from build123d import *

# Parameters (mm, degrees)
SKETCH1_W                     = 56
SKETCH1_H                     = 65
BOSS_EXTRUDE1_DEPTH           = 8
FILLET1_R                     = 3
CBORE_FOR_M4_SHCS1_AT_2_COUNT = 2
CBORE_FOR_M4_SHCS1_AT_2_PITCH = 24
M4X0_7_TAPPED_HOLE1_D         = 3.3
M4X0_7_TAPPED_HOLE1_DEPTH     = 10.1
M4X0_7_TAPPED_HOLE1_TIP       = 0.991420021


with BuildPart() as part:
    # Sketch1 → Boss-Extrude1 (new body)
    with BuildSketch(Plane.XY):
        Rectangle(SKETCH1_W, SKETCH1_H)
    extrude(amount=BOSS_EXTRUDE1_DEPTH)

    # Fillet1
    fillet1_edges = [part.edges().sort_by_distance(p)[0] for p in [
        (28, -32.5, 4),
        (-28, -32.5, 4),
        (-28, 32.5, 4),
        (28, 32.5, 4),
    ]]
    fillet(fillet1_edges, radius=FILLET1_R)

    # Sketch3 → CBORE for M4 SHCS1 (revolve, cut)
    with BuildSketch(Plane(origin=(-12, -22.5, 8), x_dir=(0, -1, 0), z_dir=(1, 0, 0))):
        Polygon((0, 0), (0, 8), (2.25, 8), (2.25, 4), (4, 4), (4, 0.025), (4.025, 0), align=None)
    cbore_for_m4_shcs1 = revolve(axis=Axis((-12, -22.5, 14.35), (0, 0, -1)), mode=Mode.SUBTRACT)

    # CBORE for M4 SHCS1 at 2: CBORE for M4 SHCS1 ×2
    with Locations(*[(i * CBORE_FOR_M4_SHCS1_AT_2_PITCH, 0, 0) for i in range(1, CBORE_FOR_M4_SHCS1_AT_2_COUNT)]):
        add(cbore_for_m4_shcs1, mode=Mode.SUBTRACT)

    # M4x0.7 Tapped Hole1
    with Locations(Plane.XY.offset(8)):
        with Locations((-23.25, -18.5), (23.25, -18.5), (23.25, 28), (-23.25, 28)):
            Hole(M4X0_7_TAPPED_HOLE1_D / 2, depth=M4X0_7_TAPPED_HOLE1_DEPTH)
            with Locations((0, 0, -(M4X0_7_TAPPED_HOLE1_DEPTH + M4X0_7_TAPPED_HOLE1_TIP / 2))):  # 118° drill point
                Cone(0, M4X0_7_TAPPED_HOLE1_D / 2, M4X0_7_TAPPED_HOLE1_TIP, mode=Mode.SUBTRACT)


solid = part.part
The model under review builds one solid part; all positions refer to its coordinate system, in mm. A direction names the side the tool comes from. Coordinates: 2 decimals unless noted, no trailing zeros. Loops run counter-clockwise (first coordinate to the right, second up) from the corner with the lowest first, then second, coordinate; pieces in that order, holes last.
(1) Tool access review of faces 4 (the cylindrical face through (-12.176, -18.504, 6.015)), 5 (the flat face through (28, 0, 4)): name each direction out of +Z, -Z, +X, -X, +Y, -Y from which nothing blocks a thin tool from reaching the whole face with its end or side.
Determined:
face 4: +Z
face 5: +Z, -Z, +X, +Y, -Y
(2) Consider section B-B, the plane x = -12. Give the boundary of the cut face in (y, z) (3 decimals).
Determined:
outline: (-32.5, 0) - (-24.75, 0) - (-24.75, 4) - (-26.5, 4) - (-26.5, 7.975) - (-26.525, 8) - (-32.5, 8) - close; (-20.25, 0) - (32.5, 0) - (32.5, 8) - (-18.475, 8) - (-18.5, 7.975) - (-18.5, 4) - (-20.25, 4) - close
(3) Consider section A-A, the plane y = -22.5. Give the boundary of the cut face in (x, z) (3 decimals), plus the area to 3 significant figures.
Determined:
outline: (-28, 0) - (-14.25, 0) - (-14.25, 4) - (-16, 4) - (-16, 7.975) - (-16.025, 8) - (-28, 8) - close; (-9.75, 0) - (9.75, 0) - (9.75, 4) - (8, 4) - (8, 7.975) - (7.975, 8) - (-7.975, 8) - (-8, 7.975) - (-8, 4) - (-9.75, 4) - close; (14.25, 0) - (28, 0) - (28, 8) - (16.025, 8) - (16, 7.975) - (16, 4) - (14.25, 4) - close
area: 348 mm2
(4) Consider section D-D, the plane x = 23.25. Give the boundary of the cut face in (y, z), plus the area to 3 significant figures.
Determined:
outline: (-32.5, 0) - (-20.15, 0) - (-20.15, 8) - (-32.5, 8) - close; (-16.85, 0) - (26.35, 0) - (26.35, 8) - (-16.85, 8) - close; (29.65, 0) - (32.5, 0) - (32.5, 8) - (29.65, 8) - close
area: 467 mm2
(5) Insertion check: P1, Ø4, axis at x = 11.5, y = -21, coming from the +Z side. The pin has a flat end and moves straight along its axis. Give the tip position at first contact, or say it passes through.
Determined:
P1: stops at z = 4
(6) Consider section C-C, the plane z = 2. Give the boundary of the cut face in (x, y).
Determined:
outline: (-28, -29.5) arc R3 ccw to (-25, -32.5) - (25, -32.5) arc R3 ccw to (28, -29.5) - (28, 29.5) arc R3 ccw to (25, 32.5) - (-25, 32.5) arc R3 ccw to (-28, 29.5) - close; hole circle Ø3.3 at (-23.25, -18.5); hole circle Ø3.3 at (-23.25, 28); hole circle Ø4.5 at (-12, -22.5); hole circle Ø4.5 at (12, -22.5); hole circle Ø3.3 at (23.25, -18.5); hole circle Ø3.3 at (23.25, 28)
(7) Draft analysis for pull direction X (two halves, no side actions). For faces 1 (the cylindrical face through (-27.14, 31.6, 4.06)), 2 (the cylindrical face through (27.14, 31.6, 4.06)), 3 (the cylindrical face through (24.466, 29.115, 3.944)), state which applies: +X half, -X half, draft (parallel to the pull), parting line (faces both ways), or undercut.
Determined:
face 1: -X half
face 2: +X half
face 3: undercut
(8) Wall thickness on L1, parallel to X at y = -22.5, z = 1.25; L2, parallel to Y at x = -23.25, z = 4; L3, parallel to Y at x = -12, z = 6.75: over which ranges is each line inside the solid? List them lowest first.
Determined:
L1: x = -28 to -14.25, -9.75 to 9.75, 14.25 to 28
L2: y = -32.5 to -20.15, -16.85 to 26.35, 29.65 to 32.5
L3: y = -32.5 to -26.5, -18.5 to 32.5
